```python
from build123d import *

# Parameters (mm, degrees)
F0_W     = 80
F0_H     = 80
F1_DEPTH = 35
F3_DEPTH = 35.001
F4_R     = 4
F5_DEPTH = 35.001


with BuildPart() as f1:
    # F0 (on Right) → F1 (new body)
    with BuildSketch(Plane.YZ):
        Rectangle(F0_W, F0_H)
    extrude(amount=F1_DEPTH)

    # F2 (on face) → F3 (cut, through all)
    with BuildSketch(Plane.YZ.offset(35)):
        with BuildLine():
            ThreePointArc((-40, 32), (-36.221541, 36.221541), (-32, 40))
            Line((-32, 40), (-40, 40))
            Line((-40, 40), (-40, 32))
        make_face()
        with BuildLine():
            ThreePointArc((-32, -40), (-36.221541, -36.221541), (-40, -32))
            Line((-40, -32), (-40, -40))
            Line((-40, -40), (-32, -40))
        make_face()
        with BuildLine():
            ThreePointArc((40, -32), (36.221541, -36.221541), (32, -40))
            Line((32, -40), (40, -40))
            Line((40, -40), (40, -32))
        make_face()
        with BuildLine():
            ThreePointArc((32, 40), (36.221541, 36.221541), (40, 32))
            Line((40, 32), (40, 40))
            Line((40, 40), (32, 40))
        make_face()
    extrude(amount=-F3_DEPTH, mode=Mode.SUBTRACT)

    # F4 (on face) → F5 (cut, through all)
    with BuildSketch(Plane(origin=(0, 0, 0), x_dir=(0, -1, 0), z_dir=(-1, 0, 0))):
        Circle(F4_R)
    extrude(amount=-F5_DEPTH, mode=Mode.SUBTRACT)


solid = f1.part
```
The model under review builds one solid part; all positions refer to its coordinate system, in mm. Give positions to 0.01 mm unless a question says otherwise; leave off trailing zeros. Write each loop counter-clockwise with the first axis right and the second up, starting at its lowest first coordinate (ties: lowest second). Pieces come first, ordered by that corner, then holes. Notation, with made-up numbers: (65, 6.5) -> (117, 6.5) arc R22 ccw to (117, 14.5) -> close; hole circle Ø3 at (4.25, 8). An arc over 180 degrees is marked (long way). Answer in a Markdown table with one row per item.
1) Add section A-A on z = 0. State the section outline as (x, y) points.
Worked answers:
| item | result |
|---|---|
| outline | (0, -40) -> (35, -40) -> (35, -4) -> (0, -4) -> close; (0, 4) -> (35, 4) -> (35, 40) -> (0, 40) -> close |
2) For L1, parallel to Z at x = 24, y = 0; L2, parallel to Y at x = 26, z = -3; L3, parallel to Y at x = 26.5, z = -1, list the stretches that pass through material, from the lowest coordinate up. Write a range as [from, to].
Worked answers:
| item | result |
|---|---|
| L1 | [-40, -4], [4, 40] |
| L2 | [-40, -2.65], [2.65, 40] |
| L3 | [-40, -3.87], [3.87, 40] |
3) Clearance check with a flat-ended pin moving along its axis: P1, Ø10, axis at y = -23.5, z = -17.5, coming from the -X side. State where the tip first meets the part, or that it passes through.
Worked answers:
| item | result |
|---|---|
| P1 | x = 0 |
4) Add section D-D on y = -34.5. State the section outline as (x, z) points.
Worked answers:
| item | result |
|---|---|
| outline | (0, -37.86) -> (35, -37.86) -> (35, 37.86) -> (0, 37.86) -> close |
5) Add section C-C on x = 25.5. State the section outline as (y, z) points, plus the area to 3 significant figures.
Worked answers:
| item | result |
|---|---|
| outline | (-40, -32) arc R51.22 ccw to (-32, -40) -> (32, -40) arc R51.22 ccw to (40, -32) -> (40, 32) arc R51.22 ccw to (32, 40) -> (-32, 40) arc R51.22 ccw to (-40, 32) -> close; hole circle Ø8 at (0, 0) |
| area | 6,230 mm² |
6) Mouldability with a two-part tool opening along Z and no side actions: class faces 1 (the flat face through (35, -1, 9)), 2 (the cylindrical face through (17.255, 0.867, -3.905)), 3 (the flat face through (17, 0, -40)) as +Z half, -Z half, draft (parallel to the pull), parting line (faces both ways), or undercut.
Worked answers:
| item | result |
|---|---|
| face 1 | draft |
| face 2 | undercut |
| face 3 | -Z half |
